Drawing for the job (mm, zero at the part's lowest x, y, z). A direction names the side the tool comes from. Coordinates: 2 decimals unless noted, no trailing zeros. Write each loop counter-clockwise with the first axis right and the second up, starting at its lowest first coordinate (ties: lowest second). Pieces come first, ordered by that corner, then holes. Notation, with made-up numbers: M 26.25,51 L 79.25,51 A14 ccw 79.25,60 Z; hole C 0.5,-25.75 d3. An arc over 180 degrees is marked long. Use CSV: the item, a comma, the result in double quotes. Start each with the question number.
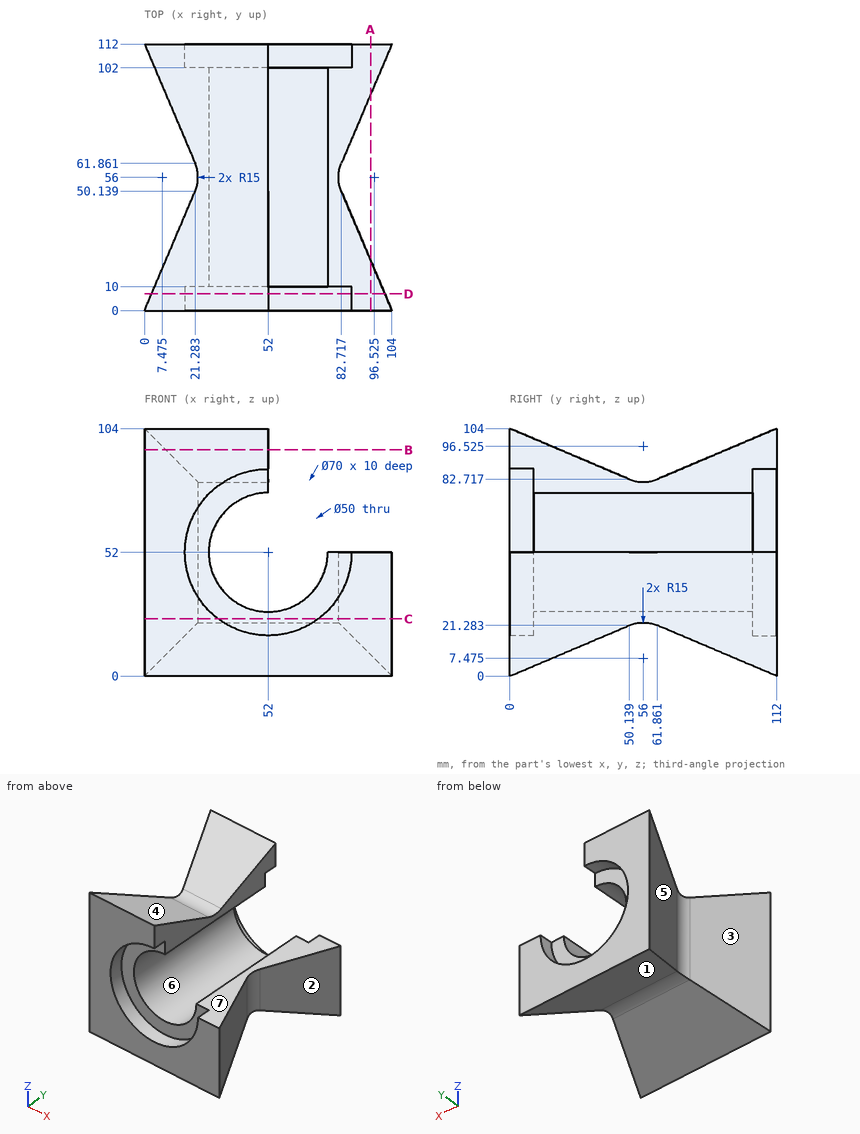
1) Band-saw the part on C-C on z = 24. List the corners of the cut face in (x, y) (1 decimal).
2) Band-saw the part on A-A on x = 95. List the corners of the cut face in (y, z).
3) Tool access for the marked faces 1, 2, 3 and 4: list every direction of +Z, -Z, +X, -X, +Y, -Y with a clear straight run to the whole face (end or side of a thin tool).
4) Two-plate mould, pull along Z, no slides. Class the marked faces 5, 6 and 7: pulls with the +Z half, pulls with the -Z half, needs draft (parallel to the pull), parting line crosses it, or undercut.
5) Band-saw the part on B-B on z = 95. List the corners of the cut face in (x, y), then the cut area to 3 significant figures.
6) Drop flat-ended pins along their axis: P1, Ø21.5, axis at x = 93.5, y = 34.5, coming from the +Z side; P2, Ø6, axis at x = 57, y = 72, coming from the +Z side (1 decimal); P3, Ø13.5, axis at y = 73, z = 93, coming from the +X side. Give the stop position or say it passes through.
7) Wall check: L1, parallel to Y at x = 94.5, z = 14.5; L2, parallel to Y at x = 31.5, z = 25; L3, parallel to Z at x = 47.5, y = 38.5. Give the ranges that are in metal, low to high. Write a range as [from, to].
8) Band-saw the part on D-D on y = 7. List the corners of the cut face in (x, z), then the cut area to 4 significant figures.
Findings below:
1,outline,"M 0,0 L 31,0 L 31,10 L 73,10 L 73,0 L 104,0 L 82.7,50.1 A15 cw 82.7,61.9 L 104,112 L 73,112 L 73,102 L 31,102 L 31,112 L 0,112 L 21.3,61.9 A15 cw 21.3,50.1 Z"
2,outline,"M 0,0 L 21.2,9 L 21.2,52 L 0,52 Z; M 90.8,9 L 112,0 L 112,52 L 90.8,52 Z"
3,face 1,"-Z, +X, -X"
3,face 2,"+Z, -Z, +X"
3,face 3,"+Z, -Z, -X"
3,face 4,"+Z, +X, -X"
4,face 5,"needs draft"
4,face 6,"undercut"
4,face 7,"pulls with the +Z half"
5,outline,"M 0,0 L 52,0 L 52,21.2 L 9,21.2 Z; M 0,112 L 9,90.8 L 52,90.8 L 52,112 Z"
5,area,"2,010 mm2"
6,P1,"stops at z = 52"
6,P2,"stops at z = 28.3"
6,P3,"stops at x = 52"
7,L1,"y = [0, 22.38], [89.62, 112]"
7,L2,"y = [10, 102]"
7,L3,"z = [16.34, 27.41], [76.59, 87.66]"
8,outline,"M 2.97,2.97 L 101.03,2.97 L 101.03,52 L 87,52 A35 cw long 52,87 L 52,101.03 L 2.97,101.03 Z"
8,area,"4,325 mm2"
